Work out the finished part from the listing and answer in its coordinate system (mm). Face numbers are marked on the shaded views. Coordinates: 2 decimals unless noted, no trailing zeros. Loops run counter-clockwise (first coordinate to the right, second up) from the corner with the lowest first, then second, coordinate; pieces in that order, holes last. Notation, with made-up numbers: (-38, 58.25) - (18, 58.25) arc R21 cw to (18, 70.25) - close; hole circle Ø5 at (32.25, 33.5). An arc over 180 degrees is marked (long way). Write each question's results on one line, items separated by ' | '. Start each with the question number.
Item 1: For a pull along Y with two mould halves and no side action, classify the marked faces 1, 2 and 3 as +Y half, -Y half, draft (parallel to the pull), parting line (faces both ways), or undercut.
Item 2: Section A-A, the plane z = 3.5 is taken. Write down the section's boundary in (x, y), plus the area to 3 significant figures.
Item 3: Section B-B, the plane y = 57.5 is taken. Write down the section's boundary in (x, z), plus the area to 3 significant figures.
Item 4: Consider probe 1 along X at (y, z) = (8, 35); probe 2 along X at (y, z) = (5, 0); probe 3 along Z at (x, y) = (104, 160.5). Determine where each line is inside the solid, lowest interval first. Write a range as [from, to].
Item 5: Each of these flat-tipped pins is pushed along its axis until it touches: pin 1 Ø8 at (y, z) = (190, 4) entering from +X; pin 2 Ø10 at (y, z) = (46, -2) entering from -X; pin 3 Ø4.5 at (y, z) = (5, 16) entering from +X; pin 4 Ø13.5 at (x, z) = (-35, -35) entering from -Y. Where does it stop, or does it pass through?
Item 6: Section C-C, the plane z = -17 is taken. Write down the section's boundary in (x, y), plus the area to 3 significant figures.
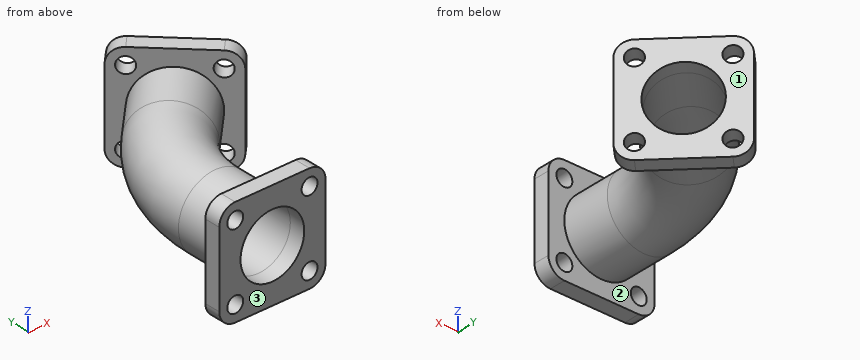
from build123d import *

# Parameters (mm, degrees)
SKETCH1_R           = 30
BOSS_EXTRUDE1_DEPTH = 15
SKETCH2_R           = 7.5
CUT_EXTRUDE1_DEPTH  = 15
SKETCH4_R           = 35
SKETCH4_R_2         = 30
BOSS_EXTRUDE2_DEPTH = 15
SKETCH7_R           = 7.5
SKETCH7_R_2         = 30
CUT_EXTRUDE2_DEPTH  = 15


with BuildPart() as part:
    # Sketch1 → Boss-Extrude1 (new body)
    with BuildSketch(Plane(origin=(0, 0, 0), x_dir=(1, 0, 0), z_dir=(0, 1, 0))):
        with BuildLine():
            Line((35, -50), (-35, -50))
            ThreePointArc((-35, -50), (-45.606601718, -45.606601718), (-50, -35))
            Line((-50, -35), (-50, 35))
            ThreePointArc((-50, 35), (-45.606601718, 45.606601718), (-35, 50))
            Line((-35, 50), (35, 50))
            ThreePointArc((35, 50), (45.606601718, 45.606601718), (50, 35))
            Line((50, 35), (50, -35))
            ThreePointArc((50, -35), (45.606601718, -45.606601718), (35, -50))
        make_face()
        with Locations(Location((0, 0, 0), (0, 0, 270))):
            Circle(SKETCH1_R, mode=Mode.SUBTRACT)
    extrude(amount=BOSS_EXTRUDE1_DEPTH)

    # Sketch2 → Cut-Extrude1 (cut)
    with BuildSketch(Plane(origin=(0, 15, 0), x_dir=(1, 0, 0), z_dir=(0, 1, 0))):
        with Locations(Location((-35, 35, 0), (0, 0, 270))):
            Circle(SKETCH2_R)
        with Locations(Location((35, 35, 0), (0, 0, 270))):
            Circle(SKETCH2_R)
        with Locations(Location((35, -35, 0), (0, 0, 270))):
            Circle(SKETCH2_R)
        with Locations(Location((-35, -35, 0), (0, 0, 270))):
            Circle(SKETCH2_R)
    extrude(amount=-CUT_EXTRUDE1_DEPTH, mode=Mode.SUBTRACT)

    # Sweep1: sweep along a path in Sketch5
    with BuildLine(Plane.XY) as sweep1_path:
        Line((0, 15), (0, 61.152236891))
        ThreePointArc((0, 61.152236891), (9.895660774, 110.901083099), (38.076118446, 153.076118446))
        Line((38.076118446, 153.076118446), (70.710678119, 185.710678119))
    # Sketch4 → Sweep1 (sweep)
    with BuildSketch(Plane(origin=(0, 15, 0), x_dir=(1, 0, 0), z_dir=(0, 1, 0))):
        Circle(SKETCH4_R)
        Circle(SKETCH4_R_2, mode=Mode.SUBTRACT)
    sweep(path=sweep1_path.line)

    # Sketch6 → Boss-Extrude2 (add)
    with BuildSketch(Plane(origin=(128.210678119, 128.210678119, 0), x_dir=(0, 0, -1), z_dir=(0.7071067811865477, 0.7071067811865474, 0))):
        with BuildLine():
            Line((35, 31.317279836), (-35, 31.317279836))
            ThreePointArc((-35, 31.317279836), (-45.606601718, 35.710678119), (-50, 46.317279836))
            Line((-50, 46.317279836), (-50, 116.317279836))
            ThreePointArc((-50, 116.317279836), (-45.606601718, 126.923881554), (-35, 131.317279836))
            Line((-35, 131.317279836), (35, 131.317279836))
            ThreePointArc((35, 131.317279836), (45.606601718, 126.923881554), (50, 116.317279836))
            Line((50, 116.317279836), (50, 46.317279836))
            ThreePointArc((50, 46.317279836), (45.606601718, 35.710678119), (35, 31.317279836))
        make_face()
    extrude(amount=BOSS_EXTRUDE2_DEPTH)

    # Sketch7 → Cut-Extrude2 (cut)
    with BuildSketch(Plane(origin=(138.817279836, 138.817279836, 0), x_dir=(0, 0, -1), z_dir=(0.7071067811865477, 0.7071067811865474, 0))):
        with Locations(Location((-35, 116.317279836, 0), (0, 0, 90))):
            Circle(SKETCH7_R)
        with Locations(Location((35, 116.317279836, 0), (0, 0, 90))):
            Circle(SKETCH7_R)
        with Locations(Location((35, 46.317279836, 0), (0, 0, 90))):
            Circle(SKETCH7_R)
        with Locations(Location((-35, 46.317279836, 0), (0, 0, 90))):
            Circle(SKETCH7_R)
        with Locations(Location((0, 81.317279836, 0), (0, 0, 90))):
            Circle(SKETCH7_R_2)
    extrude(amount=-CUT_EXTRUDE2_DEPTH, mode=Mode.SUBTRACT)


solid = part.part
Answer key:
1) face 1: +Y half | face 2: undercut | face 3: -Y half
2) outline: (-50, 0) - (-29.8, 0) - (-29.8, 61.15) arc R159.8 cw to (17.01, 174.14) - (60.25, 217.39) - (45.96, 231.67) - (35.36, 221.07) - (46.09, 210.34) - (13.45, 177.7) arc R164.82 ccw to (-34.82, 61.15) - (-34.82, 15) - (-50, 15) - close; (29.8, 0) - (50, 0) - (50, 15) - (34.82, 15) - (34.82, 61.15) arc R95.18 cw to (62.7, 128.45) - (95.34, 161.09) - (106.07, 150.36) - (116.67, 160.96) - (102.39, 175.25) - (59.14, 132.01) arc R100.2 ccw to (29.8, 61.15) - close | area: 3,170 mm^2
3) outline: circle Ø70 at (0, 0); hole circle Ø60 at (0, 0) | area: 1,020 mm^2
4) probe 1: x = [-50, -42.5], [-27.5, 27.5], [42.5, 50] | probe 2: x = [-50, -30], [30, 50] | probe 3: z = [-48.58, -38.97], [-31.03, 31.03], [38.97, 48.58]
5) pin 1: stops at x = 37.04 | pin 2: stops at x = -35 | pin 3: stops at x = 50 | pin 4: passes through
6) outline: (-50, 0) - (-24.72, 0) - (-24.72, 61.15) arc R154.72 cw to (20.6, 170.55) - (63.84, 213.8) - (45.96, 231.67) - (35.36, 221.07) - (49.08, 207.34) - (16.44, 174.71) arc R160.59 ccw to (-30.59, 61.15) - (-30.59, 15) - (-50, 15) - close; (24.72, 0) - (50, 0) - (50, 15) - (30.59, 15) - (30.59, 61.15) arc R99.41 cw to (59.71, 131.44) - (92.34, 164.08) - (106.07, 150.36) - (116.67, 160.96) - (98.8, 178.84) - (55.55, 135.6) arc R105.28 ccw to (24.72, 61.15) - close | area: 3,800 mm^2
